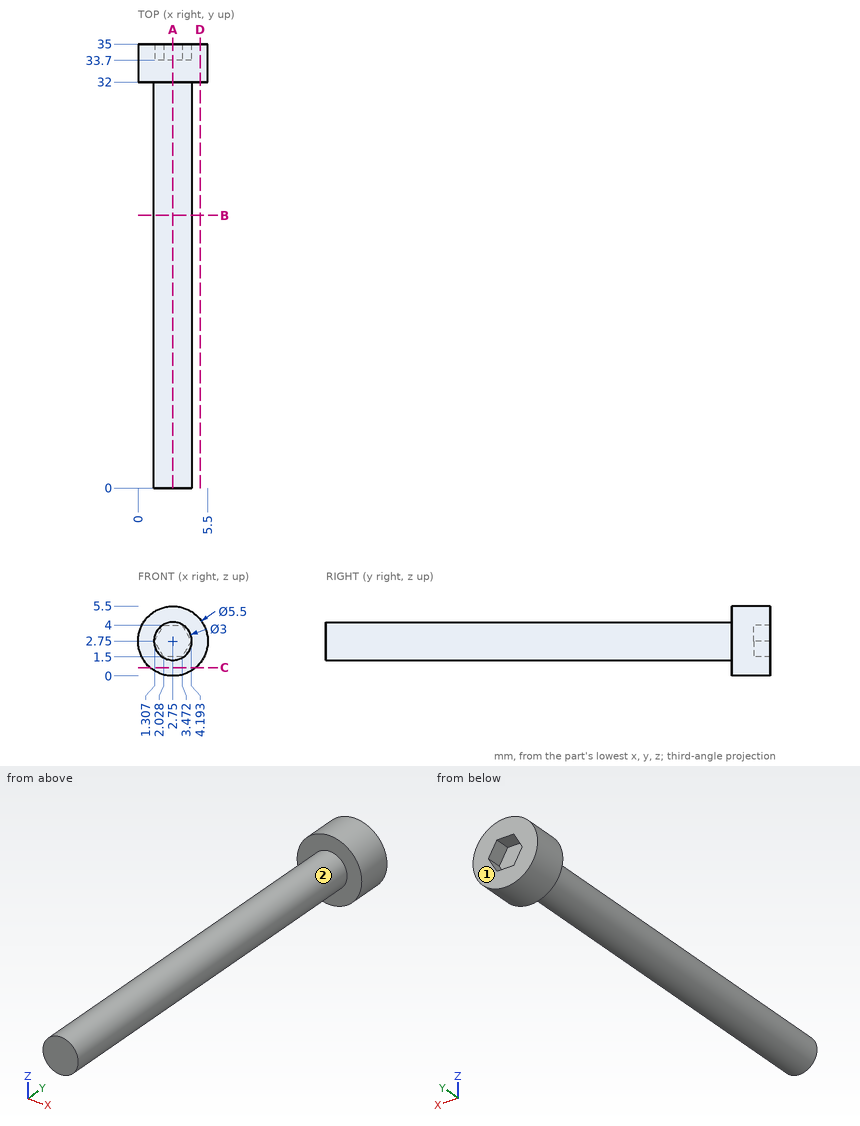
Source: three-view drawing plus pictorial views. Frame: mm from the lowest corner of the part. A direction names the side the tool comes from. Round coordinates to 2 decimals unless told otherwise and drop trailing zeros. Order: outer loops, then holes, each group sorted by start corner. A loop starts at its lowest first (then second) coordinate and runs counter-clockwise, first axis right, second up. Notation, with made-up numbers: (25, 39.5) -> (42, 39.5) arc R26 ccw to (42, 75.5) -> close; hole circle Ø3 at (62.25, -37.75). An arc over 180 degrees is marked (long way). Use one line per item in the form item = value. Start each with the question number.
1. Cut plane D-D (x = 4.9). Return the cut outline in (y, z) (1 decimal).
2. Cut plane C-C (z = 0.65). Return the cut outline in (x, y) (1 decimal).
3. Cut plane A-A (x = 2.75). Return the cut outline in (y, z), then the cut area to 3 significant figures.
4. Reachability of the marked faces 1 and 2 from +Z, -Z, +X, -X, +Y, -Y: full face, straight path, thin tool, end or side. Return the list, or none.
5. Pin query (flat end, axial travel): pin 1 Ø1.5 at (x, y) = (4.5, 3.5) entering from -Z; pin 2 Ø1 at (x, y) = (2.5, 10.5) entering from +Z; pin 3 Ø1.5 at (x, y) = (2, 12) entering from -Z. Return the tip coordinate at first contact, or that it passes through.
6. Cut plane B-B (y = 21.5). Return the cut outline in (x, z).
7. Line query: probe 1 along Y at (x, z) = (0.9, 3); probe 2 along Y at (x, z) = (1.55, 2.4); probe 3 along Z at (x, y) = (0.45, 33) (1 decimal). Output: solid intervals per line, ascending.
Solution:
q1.outline = (32, 1) -> (35, 1) -> (35, 4.5) -> (32, 4.5) -> close
q2.outline = (1, 32) -> (4.5, 32) -> (4.5, 35) -> (1, 35) -> close
q3.outline = (0, 1.25) -> (32, 1.25) -> (32, 0) -> (35, 0) -> (35, 1.5) -> (33.7, 1.5) -> (33.7, 4) -> (35, 4) -> (35, 5.5) -> (32, 5.5) -> (32, 4.25) -> (0, 4.25) -> close
q3.area = 109 mm^2
q4.face_1 = +Z, -Z, +X, -X, +Y
q4.face_2 = -Y
q5.pin_1 = 1.63
q5.pin_2 = 4.25
q5.pin_3 = 1.25
q6.outline = circle Ø3 at (2.75, 2.75)
q7.probe_1 = 32 to 35
q7.probe_2 = 0 to 33.7
q7.probe_3 = 1.2 to 4.3
